```python
from build123d import *

# Parameters (mm, degrees)
SKETCH1_W           = 150
SKETCH1_H           = 110
SKETCH1_R           = 3.2639
SKETCH1_R_2         = 1.4732
BOSS_EXTRUDE1_DEPTH = 1.6


with BuildPart() as part:
    # Sketch1 → Boss-Extrude1 (new body)
    with BuildSketch(Plane(origin=(0, 0, 0), x_dir=(1, 0, 0), z_dir=(0, 1, 0))):
        Rectangle(SKETCH1_W, SKETCH1_H)
        with Locations(Location((0, 12.7, 0), (0, 0, 270))):
            Circle(SKETCH1_R, mode=Mode.SUBTRACT)
        with Locations(Location((12.7, 0, 0), (0, 0, 270))):
            Circle(SKETCH1_R, mode=Mode.SUBTRACT)
        with Locations(Location((0, -12.7, 0), (0, 0, 270))):
            Circle(SKETCH1_R, mode=Mode.SUBTRACT)
        with Locations(Location((-12.7, 0, 0), (0, 0, 270))):
            Circle(SKETCH1_R, mode=Mode.SUBTRACT)
        with Locations(Location((-32.5, 48, 0), (0, 0, 270))):
            Circle(SKETCH1_R_2, mode=Mode.SUBTRACT)
        with Locations(Location((32.5, 48, 0), (0, 0, 270))):
            Circle(SKETCH1_R_2, mode=Mode.SUBTRACT)
        with Locations(Location((32.5, -48, 0), (0, 0, 270))):
            Circle(SKETCH1_R_2, mode=Mode.SUBTRACT)
        with Locations(Location((-32.5, -48, 0), (0, 0, 270))):
            Circle(SKETCH1_R_2, mode=Mode.SUBTRACT)
        with Locations(Location((-68, 32.5, 0), (0, 0, 270))):
            Circle(SKETCH1_R_2, mode=Mode.SUBTRACT)
        with Locations(Location((68, 32.5, 0), (0, 0, 270))):
            Circle(SKETCH1_R_2, mode=Mode.SUBTRACT)
        with Locations(Location((68, -32.5, 0), (0, 0, 270))):
            Circle(SKETCH1_R_2, mode=Mode.SUBTRACT)
        with Locations(Location((-68, -32.5, 0), (0, 0, 270))):
            Circle(SKETCH1_R_2, mode=Mode.SUBTRACT)
    extrude(amount=BOSS_EXTRUDE1_DEPTH)


solid = part.part
```
Input: part model. Units: mm. Frame: model coordinates. Give positions to 0.01 mm unless a question says otherwise; leave off trailing zeros. Order: outer loops, then holes, each group sorted by start corner. A loop starts at its lowest first (then second) coordinate and runs counter-clockwise, first axis right, second up. Notation, with made-up numbers: (32, -33.5) -> (72, -33.5) arc R11 ccw to (72, -29.5) -> close; hole circle Ø10 at (-25.5, 0). An arc over 180 degrees is marked (long way). Write each question's results on one line, items separated by ' | '. Start each with the question number.
Item 1: Line query: line 1 (X direction, y = 1.15, z = -32.5); line 2 (X direction, y = 1, z = -48); line 3 (Z direction, x = -68, y = 0.9). Output: solid intervals per line, ascending.
Item 2: Cut plane A-A on x = -12.7. Return the cut outline in (y, z).
Item 3: Cut plane B-B on z = 0. Return the cut outline in (x, y), then the cut area to 3 significant figures.
Item 4: Contact query for a flat-ended pin moving along its axis: P1, Ø8, axis at x = -5, z = -0.5, coming from the -Y side. Output: stop coordinate, or through.
Item 5: Mould query, pull axis Z, two halves, no side actions, for faces 1 (the flat face through (-1, 0, -1)), 2 (the cylindrical face through (32.56, 0.79, -49.47)). Classes: pulls with the +Z half, pulls with the -Z half, needs draft (parallel to the pull), parting line crosses it, or undercut.
Item 6: Cut plane C-C on z = 12.7. Return the cut outline in (x, y).
Established:
1) line 1: -75 to -69.47, -66.53 to 66.53, 69.47 to 75 | line 2: -75 to -33.97, -31.03 to 31.03, 33.97 to 75 | line 3: -55 to -33.97, -31.03 to 31.03, 33.97 to 55
2) outline: (0, -55) -> (1.6, -55) -> (1.6, -3.26) -> (0, -3.26) -> close; (0, 3.26) -> (1.6, 3.26) -> (1.6, 55) -> (0, 55) -> close
3) outline: (-75, 0) -> (-15.96, 0) -> (-15.96, 1.6) -> (-75, 1.6) -> close; (-9.44, 0) -> (9.44, 0) -> (9.44, 1.6) -> (-9.44, 1.6) -> close; (15.96, 0) -> (75, 0) -> (75, 1.6) -> (15.96, 1.6) -> close | area: 219 mm^2
4) P1: y = 0
5) face 1: needs draft | face 2: undercut
6) outline: (-75, 0) -> (-3.26, 0) -> (-3.26, 1.6) -> (-75, 1.6) -> close; (3.26, 0) -> (75, 0) -> (75, 1.6) -> (3.26, 1.6) -> close
